from build123d import *

# Parameters (mm, degrees)
F0_W     = 393.7
F0_H     = 95.25
F1_DEPTH = 133.35
F2_W     = 381
F2_H     = 127
F3_DEPTH = 88.9
F4_W     = 50.8
F4_H     = 88.9
F5_DEPTH = 406.4
F6_W     = 381
F6_H     = 25.4
F7_DEPTH = 25.4


with BuildPart() as f1:
    # F0 (on Front) → F1 (new body)
    with BuildSketch(Plane.XZ):
        Rectangle(F0_W, F0_H)
    extrude(amount=F1_DEPTH)

    # F2 (on face) → F3 (cut)
    with BuildSketch(Plane.XY.offset(47.625)):
        with Locations((0, -63.5)):
            Rectangle(F2_W, F2_H)
    extrude(amount=-F3_DEPTH, mode=Mode.SUBTRACT)

    # F4 (on face) → F5 (cut)
    with BuildSketch(Plane(origin=(-196.85, 0, 0), x_dir=(0, -1, 0), z_dir=(-1, 0, 0))):
        with Locations((25.4, 3.175)):
            Rectangle(F4_W, F4_H)
    extrude(amount=-F5_DEPTH, mode=Mode.SUBTRACT)

    # F6 (on face) → F7 (cut)
    with BuildSketch(Plane(origin=(0, -127, 0), x_dir=(-1, 0, 0), z_dir=(0, 1, 0))):
        with Locations((0, 34.925)):
            Rectangle(F6_W, F6_H)
    extrude(amount=-F7_DEPTH, mode=Mode.SUBTRACT)


solid = f1.part
CAD build for the part. Positions are in the model's coordinates, mm. A direction names the side the tool comes from. Round coordinates to 2 decimals unless told otherwise and drop trailing zeros. Order: outer loops, then holes, each group sorted by start corner. A loop starts at its lowest first (then second) coordinate and runs counter-clockwise, first axis right, second up. Notation, with made-up numbers: (85, 6.5) -> (116, 6.5) arc R22 ccw to (116, 20.5) -> close; hole circle Ø5 at (86.25, 38.5). An arc over 180 degrees is marked (long way). Write item = value, one per line. Start each with the question number.
(1) Cut at C-C, the plane z = -31. List the corners of the cut face in (x, y), then the cut area to 3 significant figures.
(2) Cut at D-D, the plane x = -40. List the corners of the cut face in (y, z) (3 decimals).
(3) Which spindle directions (+Z, -Z, +X, -X, +Y, -Y) get a long thin tool onto all of the face, cutting with end or side? Do faces 1 (the flat face through (-3, -66, -47.625)), 2 (the flat face through (-3, -127, -9)). Say none if no direction does.
(4) Cut at A-A, the plane y = -80. List the corners of the cut face in (x, z) (3 decimals).
(5) Probe line 1 (X direction, y = -126, z = -12); line 2 (Z direction, x = -128, y = -19.5) (3 decimals); line 3 (Y direction, x = 38.5, z = -34). List the from-to ranges inside material, lowest first. Write a range as [from, to].
(6) Pin check, flat tips, straight feed: P1, Ø12, axis at x = -45.5, z = 19, coming from the +Y side; P2, Ø1.9, axis at x = 31.5, y = -129, coming from the +Z side (3 decimals); P3, Ø5, axis at x = 114, y = -81.5, coming from the +Z side (3 decimals). Stop position of each tip, or through.
(7) Pull direction X, two halves, no side cores. Call faces 3 (the flat face through (-196.85, -81, -1)), 4 (the flat face through (190.5, -93, 4)), 5 (the flat face through (-3, -133.35, -10)), 6 (the flat face through (-190.5, -93, 4)): released by +X, released by -X, zero draft, split by the parting line, or undercut.
(8) Cut at B-B, the plane z = 38.5. List the corners of the cut face in (x, y), then the cut area to 3 significant figures.
Model answer:
q1.outline = (-196.85, -133.35) -> (196.85, -133.35) -> (196.85, -50.8) -> (190.5, -50.8) -> (190.5, -127) -> (-190.5, -127) -> (-190.5, -50.8) -> (-196.85, -50.8) -> close
q1.area = 3,470 mm2
q2.outline = (-133.35, -47.625) -> (0, -47.625) -> (0, -41.275) -> (-127, -41.275) -> (-127, 22.225) -> (-133.35, 22.225) -> close
q3.face_1 = -Z, +X, -X, +Y, -Y
q3.face_2 = +Z, +Y
q4.outline = (-196.85, -47.625) -> (196.85, -47.625) -> (196.85, 47.625) -> (190.5, 47.625) -> (190.5, -41.275) -> (-190.5, -41.275) -> (-190.5, 47.625) -> (-196.85, 47.625) -> close
q5.line_1 = [-196.85, -190.5], [190.5, 196.85]
q5.line_2 = [-47.625, -41.275]
q5.line_3 = [-133.35, -127]
q6.P1 = -127
q6.P2 = 22.225
q6.P3 = -41.275
q7.face_3 = released by -X
q7.face_4 = undercut
q7.face_5 = zero draft
q7.face_6 = undercut
q8.outline = (-196.85, -133.35) -> (-190.5, -133.35) -> (-190.5, -50.8) -> (-196.85, -50.8) -> close; (190.5, -133.35) -> (196.85, -133.35) -> (196.85, -50.8) -> (190.5, -50.8) -> close
q8.area = 1,050 mm2
